Autodesk Inventor part; units mm, degrees
ref_plane "Work Plane1" through (-56.3599, 0, 22) normal (0, 0, -1) x (-1, 0, 0)
ref_plane "YZ Plane" through (0, 0, 0) normal (1, 0, 0) x (0, 1, 0)
ref_plane "XZ Plane" through (0, 0, 0) normal (0, 1, 0) x (-1, 0, 0)
ref_plane "Work Plane1" through (-56.3599, 0, 22) normal (0, 0, -1) x (-1, 0, 0)
sketch "Sketch1" plane through (-56.3599, 0, 22) normal (0, 0, -1) x (-1, 0, 0)
  line L0 (-4.0299, -0.3538) -> (-2.2322, 1.4439) construction
  arc A0 (-1.4439, 2.2322) -> (-2.2322, 1.4439) centre (-0.9299, 0.9299) ccw construction
  line L1 (-1.4439, 2.2322) -> (0.3538, 4.0299) construction
  line L2 (-37.8299, 42.8299) -> (-37.8299, 37.8299) construction
  line L3 (-37.8299, 37.8299) -> (-42.9208, 37.8299) construction
  line L4 (-37.8299, 42.2137) -> (-37.8299, 45.8299) construction
  line L5 (-37.8299, 45.8299) -> (-4.0299, 45.8299) construction
  line L6 (-4.0299, 45.8299) -> (-4.0299, 42.2137) construction
  line L7 (-4.0299, 4.0299) -> (0.3538, 4.0299)
  circle A1 centre (-20.9299, 20.9299) radius 17.5
  line L8 (-20.9299, 58.9723) -> (17.1124, 20.9299) construction
  line L9 (17.1124, 20.9299) -> (-20.9299, -17.1124) construction
  line L10 (-20.9299, -17.1124) -> (-58.9723, 20.9299) construction
  line L11 (-58.9723, 20.9299) -> (-20.9299, 58.9723) construction
  line L12 (-20.9299, 58.9723) -> (-20.9299, -17.1124) construction
  line L13 (17.1124, 20.9299) -> (-58.9723, 20.9299) construction
  line L14 (-20.9299, 58.9723) -> (32.8701, 58.9723) construction
  line L15 (-43.4299, 43.4299) -> (1.5701, 43.4299) construction
  line L16 (1.5701, 43.4299) -> (1.5701, -1.5701) construction
  line L17 (1.5701, -1.5701) -> (-43.4299, -1.5701) construction
  line L18 (-43.4299, -1.5701) -> (-43.4299, 43.4299) construction
  line L19 (-43.4299, 43.4299) -> (1.5701, -1.5701) construction
  line L20 (1.5701, 43.4299) -> (-43.4299, -1.5701) construction
  line L21 (-43.4299, 5.3876) -> (-43.4299, 36.4723)
  line L22 (-43.4299, 36.4723) -> (-36.4723, 43.4299)
  line L23 (-36.4723, 43.4299) -> (-5.3876, 43.4299)
  line L24 (-5.3876, 43.4299) -> (1.5701, 36.4723)
  line L25 (1.5701, 36.4723) -> (1.5701, 5.3876)
  line L26 (1.5701, 5.3876) -> (-5.3876, -1.5701)
  line L27 (-5.3876, -1.5701) -> (-36.4723, -1.5701)
  line L28 (-36.4723, -1.5701) -> (-43.4299, 5.3876)
  line L29 (-4.0299, 42.2137) -> (-37.8299, 42.2137)
  line L30 (-4.0299, -0.3538) -> (-4.0299, 4.0299)
  circle A2 centre (-20.9299, 20.9299) radius 1.5
  line L31 (-10.9299, 10.9299) -> (-30.9299, 10.9299) construction
  line L32 (-30.9299, 10.9299) -> (-30.9299, 30.9299) construction
  line L33 (-30.9299, 30.9299) -> (-10.9299, 30.9299) construction
  line L34 (-10.9299, 30.9299) -> (-10.9299, 10.9299) construction
  line L35 (-10.9299, 10.9299) -> (-30.9299, 30.9299) construction
  line L36 (-30.9299, 10.9299) -> (-10.9299, 30.9299) construction
  circle A3 centre (-30.9299, 30.9299) radius 1.4
  circle A4 centre (-30.9299, 10.9299) radius 1.4
  circle A5 centre (-10.9299, 10.9299) radius 1.4
  line L37 (-45.8299, 37.8299) -> (-42.0723, 37.8299) construction
  line L38 (-42.1723, 37.7299) -> (-45.8299, 37.7299)
  line L39 (-45.8299, 37.7299) -> (-45.8299, 4.1299)
  line L40 (-45.8299, 4.1299) -> (-42.1723, 4.1299)
  line L41 (-42.1723, 4.1299) -> (-42.1723, 37.7299)
  line L42 (-45.8299, 4.0299) -> (-42.0723, 4.0299) construction
  line L43 (-45.8299, 37.8299) -> (-42.0723, 37.8299)
  line L44 (-37.7299, 45.8299) -> (-4.1299, 45.8299)
  line L45 (-4.1299, 45.8299) -> (-4.1299, 42.1723)
  line L46 (-4.1299, 42.1723) -> (-37.7299, 42.1723)
  line L47 (-37.7299, 42.1723) -> (-37.7299, 45.8299)
  line L48 (0.4701, 37.8299) -> (0.4701, 4.0299) construction
  line L49 (0.4701, 4.0299) -> (3.9701, 4.0299) construction
  line L50 (3.9701, 37.8299) -> (3.9701, 4.0299) construction
  line L51 (0.4701, 37.8299) -> (3.9701, 37.8299) construction
  line L52 (-45.8299, -3.9701) -> (-4.0299, -3.9701) construction
  line L53 (0.3124, 37.7299) -> (3.9701, 37.7299)
  line L54 (3.9701, 37.7299) -> (3.9701, 4.1299)
  line L55 (3.9701, 4.1299) -> (0.3124, 4.1299)
  line L56 (0.3124, 4.1299) -> (0.3124, 37.7299)
  line L57 (-4.1713, -0.3538) -> (-37.7299, -0.3538)
  line L58 (-37.7299, -0.3538) -> (-37.7299, -3.9701)
  line L59 (-37.7299, -3.9701) -> (-4.1713, -3.9701)
  line L60 (-4.1713, -3.9701) -> (-4.1713, -0.3538)
  point P0 (-37.8299, 4.0299)
  dimension "d18" = 53.8
  dimension "d19" = 45
  dimension "d20" = 53.8
  dimension "d21" = 45
  dimension "d22" = 45
  dimension "d30" = 20
  dimension "d31" = 20
  dimension "d32" = 2.8
  dimension "d33" = 2.8
  dimension "d34" = 2.8
  dimension "d35" = 3
  dimension "d36" = 0.1
  dimension "d37" = 0.1
  dimension "d38" = 0.1
  dimension "d39" = 0.1
extrude "Extrusion1" add sketch "Sketch1" along normal blind 6 contours L30 L26 L57 L28 L41 L22 L46 L24 L56 L7 | L7 L26 L30 | L56 L24 L25 L26 | L26 L25 L24 L53 L54 L55 | L60 L59 L58 L57 L28 L27 L26 | L26 L27 L28 L57 | L46 L22 L29 L24 | L24 L29 L45 | L40 L39 L38 L22 L21 L28 | L28 L21 L22 L41 | L29 L22 L23 L24 | L24 L23 L22 L29 L47 L44 L45 | L47 L29 L22 | A1 | A2 | A3 | A4 | A5
sketch "Skizze4" plane through (-56.3599, 0, 16) normal (0, 0, -1) x (-1, 0, 0)
  line L0 (-37.7299, 42.1723) -> (-42.1723, 37.7299)
  line L1 (-42.1723, 37.7299) -> (-45.8299, 37.7299)
  line L2 (-45.8299, 37.7299) -> (-45.8299, 4.1299) construction
  line L3 (-45.8299, 4.1299) -> (-42.1723, 4.1299)
  line L4 (-42.1723, 4.1299) -> (-37.6885, -0.3538)
  line L5 (-37.6885, -0.3538) -> (-37.7299, -0.3538)
  line L6 (-37.7299, -0.3538) -> (-37.7299, -3.9701)
  line L7 (-37.7299, -3.9701) -> (-4.1713, -3.9701) construction
  line L8 (-4.1713, -3.9701) -> (-4.1713, -0.3538)
  line L9 (-4.1713, -0.3538) -> (0.3124, 4.1299)
  line L10 (0.3124, 4.1299) -> (3.9701, 4.1299)
  line L11 (3.9701, 4.1299) -> (3.9701, 37.7299) construction
  line L12 (3.9701, 37.7299) -> (0.3124, 37.7299)
  line L13 (0.3124, 37.7299) -> (-4.1299, 42.1723)
  line L14 (-4.1299, 42.1723) -> (-4.1299, 45.8299)
  line L15 (-4.1299, 45.8299) -> (-37.7299, 45.8299) construction
  line L16 (-37.7299, 45.8299) -> (-37.7299, 42.1723)
  line L17 (-37.9299, 46.0299) -> (-3.9299, 46.0299) construction
  line L18 (-3.9299, 46.0299) -> (-3.9299, 42.2551)
  line L19 (-3.9299, 42.2551) -> (0.3953, 37.9299)
  line L20 (0.3953, 37.9299) -> (4.1701, 37.9299)
  line L21 (4.1701, 37.9299) -> (4.1701, 3.9299) construction
  line L22 (4.1701, 3.9299) -> (0.3953, 3.9299)
  line L23 (0.3953, 3.9299) -> (-3.9713, -0.4367)
  line L24 (-3.9713, -0.4367) -> (-3.9713, -4.1701)
  line L25 (-3.9713, -4.1701) -> (-37.9299, -4.1701) construction
  line L26 (-37.9299, -4.1701) -> (-37.9299, -0.3953)
  line L27 (-37.9299, -0.3953) -> (-42.2551, 3.9299)
  line L28 (-42.2551, 3.9299) -> (-46.0299, 3.9299)
  line L29 (-46.0299, 3.9299) -> (-46.0299, 37.9299) construction
  line L30 (-46.0299, 37.9299) -> (-42.2551, 37.9299)
  line L31 (-42.2551, 37.9299) -> (-37.9299, 42.2551)
  line L32 (-37.9299, 42.2551) -> (-37.9299, 46.0299)
  line L33 (-45.8299, 37.7299) -> (-45.8299, 37.9299)
  line L34 (-4.1299, 45.8299) -> (-37.7299, 45.8299)
  line L35 (-37.7299, 45.8299) -> (-37.9299, 45.8299)
  line L36 (-4.1299, 45.8299) -> (-3.9299, 45.8299)
  line L37 (3.9701, 37.7299) -> (3.9701, 37.9299)
  line L38 (3.9701, 4.1299) -> (3.9701, 37.7299)
  line L39 (3.9701, 4.1299) -> (3.9701, 3.9299)
  line L40 (-4.1713, -3.9701) -> (-3.9713, -3.9701)
  line L41 (-37.7299, -3.9701) -> (-37.9299, -3.9701)
  line L42 (-45.8299, 4.1299) -> (-45.8299, 3.9299)
  point P0 (-56.3599, 0)
  dimension "d40" = 0.2
extrude "IM_offset" add sketch "Skizze4" against normal up to surface (6 mm away)
ref_plane "Arbeitsebene5" through (-35.4299, 3.9299, 22) normal (-1, 0, 0) x (0, 0, 1)
ref_plane "Arbeitsebene6" through (-18.4299, 20.9299, 22) normal (0, 1, 0) x (-1, 0, 0)
properties part number "20_Cube_Insert_Electronics_v3"
Geometry check sheet. Reference: the model listing, model coordinates, mm. A direction names the side the tool comes from. Round coordinates to 2 decimals unless told otherwise and drop trailing zeros. Write each loop counter-clockwise with the first axis right and the second up, starting at its lowest first coordinate (ties: lowest second). Pieces come first, ordered by that corner, then holes. Notation, with made-up numbers: (-19.5, 55.5) - (9.5, 55.5) arc R12 cw to (9.5, 61.5) - close; hole circle Ø2 at (-39.5, 80). An arc over 180 degrees is marked (long way). One line per item, written item: value.
1. Cross-section at B-B on x = -17.5. Record the boundary of the cut face in (y, z), and give its area (3 significant figures).
The answers:
outline: (0.53, 16) - (41.33, 16) - (41.33, 22) - (0.53, 22) - close
area: 245 mm^2
2. Depth check by flat-ended pin: pin 1 Ø1.1 at (x, z) = (-13, 19) entering from -Y; pin 2 Ø1.8 at (y, z) = (-3, 19) entering from -X; pin 3 Ø1.8 at (x, z) = (-59.5, 20) entering from +Y. Enter the tip coordinate at first touch or a pass-through.
The answers:
pin 1: stops at y = 3.93
pin 2: stops at x = -52.39
pin 3: stops at y = 37.93
3. Scan lines: L1, parallel to X at y = 42.5, z = 20.9; L2, parallel to Y at x = -57, z = 21.3; L3, parallel to Y at x = -54.5, z = 17.45. Record each from-to range of solid material in increasing order.
The answers:
L1: x = -52.43 to -18.43
L2: y = 3.93 to 37.93
L3: y = 1.67 to 40.19
4. Set-up check for faces 1 (the face through (-59, 3.93, 19)), 2 (the face through (-18.43, 44, 19)), 3 (the face through (-12, 3.93, 19)): record each of +Z, -Z, +X, -X, +Y, -Y from which the full face is reachable in a straight line by a thin tool's end or side.
The answers:
face 1: +Z, -Z, -X, -Y
face 2: +Z, -Z, +X, +Y
face 3: +Z, -Z, +X, -Y
5. Cross-section at A-A on z = 18.5. Record the boundary of the cut face in (x, y).
The answers:
outline: (-60.33, 3.93) - (-56.76, 3.93) - (-52.39, -0.44) - (-52.39, -3.97) - (-18.43, -3.97) - (-18.43, -0.4) - (-14.1, 3.93) - (-10.53, 3.93) - (-10.53, 37.93) - (-14.1, 37.93) - (-18.43, 42.26) - (-18.43, 45.83) - (-52.43, 45.83) - (-52.43, 42.26) - (-56.76, 37.93) - (-60.33, 37.93) - close
